Drawing for the job (mm, zero at the part's lowest x, y, z). A direction names the side the tool comes from. Round coordinates to 2 decimals unless told otherwise and drop trailing zeros. Write each loop counter-clockwise with the first axis right and the second up, starting at its lowest first coordinate (ties: lowest second). Pieces come first, ordered by that corner, then holes. Notation, with made-up numbers: (38.25, 52) - (46.25, 52) arc R18 ccw to (46.25, 71) - close; hole circle Ø2 at (-6.5, -9). An arc over 180 degrees is marked (long way). One line per question, with ' | ' between items.
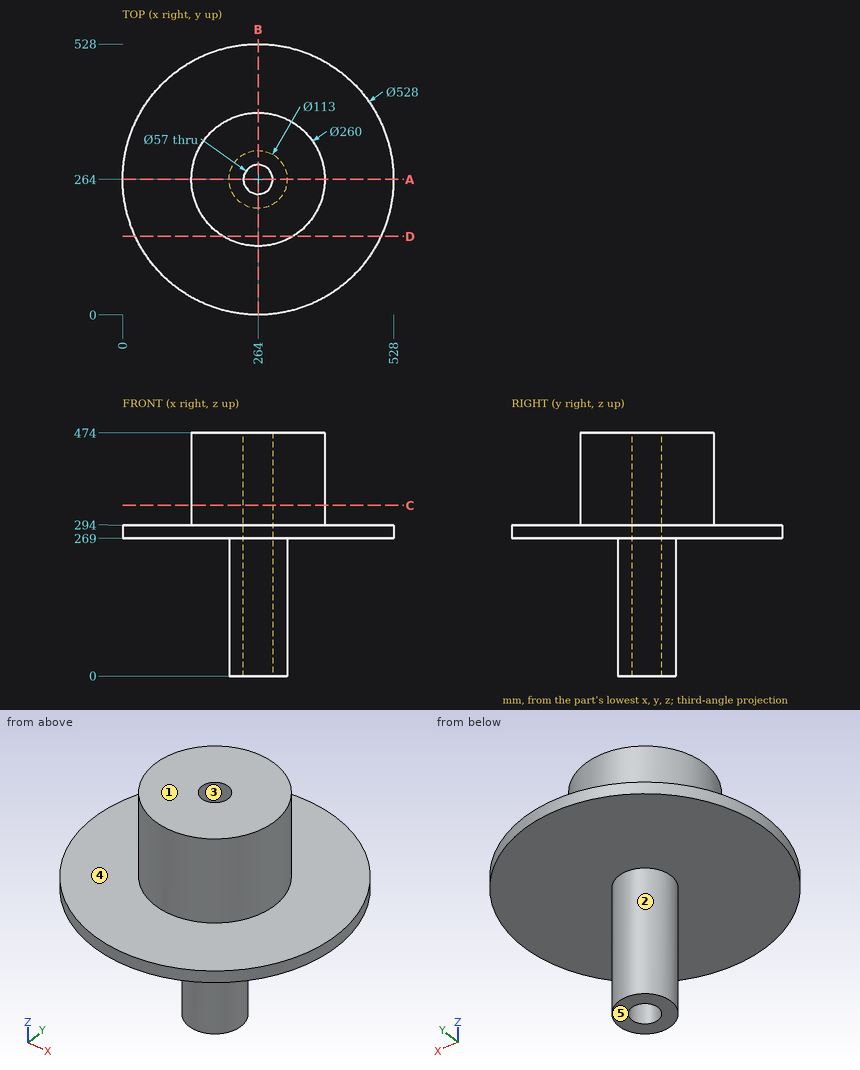
Q1. Saw through at C-C, the plane z = 332.5. List the corners of the cut face in (x, y).
Found:
outline: circle Ø260 at (264, 264); hole circle Ø57 at (264, 264)
Q2. Saw through at D-D, the plane y = 153. List the corners of the cut face in (x, z), then the cut area to 3 significant figures.
Found:
outline: (24.47, 269) - (503.53, 269) - (503.53, 294) - (331.67, 294) - (331.67, 474) - (196.33, 474) - (196.33, 294) - (24.47, 294) - close | area: 36,300 mm^2
Q3. Pull direction X, two halves, no side cores. Call the marked faces 1, 2 and 3: +X half, -X half, draft (parallel to the pull), parting line (faces both ways), or undercut.
Found:
face 1: draft | face 2: parting line | face 3: undercut
Q4. Drill centre lines: L1, parallel to X at y = 267, z = 56.5; L2, parallel to Y at x = 264, z = 370; L3, parallel to Z at x = 152.5, y = 236. Where is each one in solid material? Low to high. Write a range as from..to.
Found:
L1: 207.58..235.66, 292.34..320.42 | L2: 134..235.5, 292.5..394 | L3: 269..474
Q5. Saw through at A-A, the plane y = 264. List the corners of the cut face in (x, z).
Found:
outline: (0, 269) - (207.5, 269) - (207.5, 0) - (235.5, 0) - (235.5, 474) - (134, 474) - (134, 294) - (0, 294) - close; (292.5, 0) - (320.5, 0) - (320.5, 269) - (528, 269) - (528, 294) - (394, 294) - (394, 474) - (292.5, 474) - close
Q6. Which spindle directions (+Z, -Z, +X, -X, +Y, -Y) get a long thin tool onto all of the face, cutting with end or side? Do the marked faces 4 and 5. Say none if no direction does.
Found:
face 4: +Z | face 5: -Z, +X, -X, +Y, -Y
Q7. Drop flat-ended pins along their axis: pin 1 (12 mm diameter, centred on y = 288, z = 156.5, fed in from -X); pin 2 (3 mm diameter, centred on x = 125, y = 365.5, fed in from -Z); pin 3 (1 mm diameter, centred on x = 230.5, y = 95.5, fed in from +Z). Give the stop position or say it passes through.
Found:
pin 1: x = 210.44 | pin 2: z = 269 | pin 3: z = 294
